```python
from build123d import *

# Parameters (mm, degrees)
SKETCH4_R = 0.5
SKETCH5_R = 0.5
SKETCH6_R = 0.5


with BuildPart() as part:
    # Sweep1: sweep along a path in Sketch1
    with BuildLine(Plane.XY) as sweep1_path:
        Line((0, 0), (22, 0))
        ThreePointArc((22, 0), (22.707106781, -0.292893219), (23, -1))
        Line((23, -1), (23, -4))
    # Sketch4 → Sweep1 (sweep)
    with BuildSketch(Plane(origin=(0, 0, 0), x_dir=(0, 0, -1), z_dir=(1, 0, 0))):
        Circle(SKETCH4_R)
    sweep(path=sweep1_path.line)

    # Sweep2: sweep along a path in Sketch3
    with BuildLine(Plane(origin=(0, 0, 0), x_dir=(-1, 0, 0), z_dir=(0, 0.988012034, 0.15437688))) as sweep2_path:
        ThreePointArc((0, -24.291202111), (0.707106781, -23.998308892), (1, -23.291202111))
        Line((1, -23.291202111), (1, -1))
        ThreePointArc((1, -1), (0.707106781, -0.292893219), (0, 0))
    # Sketch5 → Sweep2 (sweep)
    with BuildSketch(Plane.ZY):
        Circle(SKETCH5_R)
    sweep(path=sweep2_path.line)

    # Sweep3: sweep along a path in Sketch2
    with BuildLine(Plane.XY.offset(-24)) as sweep3_path:
        Line((0, 3.75), (22, 3.75))
        ThreePointArc((22, 3.75), (22.707106781, 3.457106781), (23, 2.75))
        Line((23, 2.75), (23, -4))
    # Sketch6 → Sweep3 (sweep)
    with BuildSketch(Plane(origin=(0, 0, 0), x_dir=(0, 0, -1), z_dir=(1, 0, 0))):
        with Locations((24, 3.75)):
            Circle(SKETCH6_R)
    sweep(path=sweep3_path.line)


solid = part.part
```
Design review of the part built by this model. Coordinates are the model's own, in mm. A direction names the side the tool comes from. Give positions to 0.01 mm unless a question says otherwise; leave off trailing zeros. Write each loop counter-clockwise with the first axis right and the second up, starting at its lowest first coordinate (ties: lowest second). Pieces come first, ordered by that corner, then holes. Notation, with made-up numbers: (-33, 21) - (4, 21) arc R29 cw to (4, 48) - close; hole circle Ø5 at (43, -30). An arc over 180 degrees is marked (long way). Return JSON: item names as keys, results as strings. Group by question number.
(1) We need section B-B, the plane y = -1.5. Give the boundary of the cut face in (x, z).
(2) To check wall thickness, follow probe 1 along X at (y, z) = (0.5, -2); probe 2 along Z at (x, y) = (20.25, 3.5); probe 3 along Z at (x, y) = (1.75, -0.25). State the ranges of each line that lie inside material, in increasing order.
(3) Mouldability with a two-part tool opening along Z and no side actions: class faces 4 (the cylindrical face through (23.4, -0.7, -24.3)), 5 (the flat face through (23, -4, 0)), 6 (the cylindrical face through (11.154, 3.558, -24.462)) as +Z half, -Z half, draft (parallel to the pull), parting line (faces both ways), or undercut.
(4) Insertion check: pin 1 (1.5 mm diameter, centred on x = 5.5, y = 3, fed in from +Z); pin 2 (1.5 mm diameter, centred on x = 13, y = 0.5, fed in from +Z); pin 3 (3 mm diameter, centred on x = 2, z = -21.5, fed in from +Y). Each pin has a flat end and moves straight along its axis. Give the tip position at first contact, or say it passes through.
(5) Machinability: for faces 1 (the cylindrical face through (23.496, -2.521, 0.065)), 2 (the flat face through (23, -4, -24)), 3 (the cylindrical face through (11.154, -0.488, 0.108)), which of the approach directions +Z, -Z, +X, -X, +Y, -Y give a long, thin tool a straight path to every point of the face, cutting with its end or side? Answer none if there is none.
(6) We need section A-A, the plane x = 21. Give the boundary of the cut face in (y, z), then the cut area to 3 significant figures.
Reported:
{
 "1": {"outline": "circle Ø1 at (23, -24); circle Ø1 at (23, 0)"},
 "2": {"probe 1": "x = -1.46 to -0.54", "probe 2": "z = -24.43 to -23.57", "probe 3": "z = -0.43 to 0.43"},
 "3": {"face 4": "undercut", "face 5": "draft", "face 6": "parting line"},
 "4": {"pin 1": "stops at z = -23.5", "pin 2": "stops at z = 0.5", "pin 3": "passes through"},
 "5": {"face 1": "-Y", "face 2": "+Z, -Z, +X, -X, -Y", "face 3": "none"},
 "6": {"outline": "circle Ø1 at (0, 0); circle Ø1 at (3.75, -24)", "area": "1.57 mm2"}
}
